```python
from build123d import *

# Parameters (mm, degrees)
SKETCH2_R                            = 2.0193
BOSS_EXTRUDE1_DEPTH                  = 304.8
F_10_32_TAPPED_HOLE2_D               = 4.0386
F_10_32_TAPPED_HOLE2_DEPTH           = 16.34744
F_10_32_TAPPED_HOLE2_TIP             = 1.213317848
F_10_32_TAPPED_HOLE2_ON_FACE_2_D     = 4.0386
F_10_32_TAPPED_HOLE2_ON_FACE_2_DEPTH = 16.34744
F_10_32_TAPPED_HOLE2_ON_FACE_2_TIP   = 1.213317848


with BuildPart() as part:
    # Sketch2 → Boss-Extrude1 (new, symmetric)
    with BuildSketch(Plane.XY):
        with BuildLine():
            ThreePointArc((0.741687758, 5.071047688), (0, 5.125000037), (-0.741687758, 5.071047688))
            Line((-0.741687758, 5.071047688), (-4.020812242, 3.177844283))
            ThreePointArc((-4.020812242, 3.177844283), (-4.438380226, 2.562500019), (-4.7625, 1.893203404))
            Line((-4.7625, 1.893203404), (-4.7625, -1.893203404))
            ThreePointArc((-4.7625, -1.893203404), (-4.438380226, -2.562500019), (-4.020812242, -3.177844283))
            Line((-4.020812242, -3.177844283), (-0.741687758, -5.071047688))
            ThreePointArc((-0.741687758, -5.071047688), (0, -5.125000037), (0.741687758, -5.071047688))
            Line((0.741687758, -5.071047688), (4.020812242, -3.177844283))
            ThreePointArc((4.020812242, -3.177844283), (4.438380226, -2.562500019), (4.7625, -1.893203404))
            Line((4.7625, -1.893203404), (4.7625, 1.893203404))
            ThreePointArc((4.7625, 1.893203404), (4.438380226, 2.562500019), (4.020812242, 3.177844283))
            Line((4.020812242, 3.177844283), (0.741687758, 5.071047688))
        make_face()
        with Locations(Location((0, 0, 0), (0, 0, 180))):
            Circle(SKETCH2_R, mode=Mode.SUBTRACT)
    extrude(amount=BOSS_EXTRUDE1_DEPTH, both=True)

    # #10-32 Tapped Hole2
    with Locations(Plane(origin=(0, 0, -304.8), x_dir=(-1, 0, 0), z_dir=(0, 0, -1))):
        with Locations((0, 0)):
            Hole(F_10_32_TAPPED_HOLE2_D / 2, depth=F_10_32_TAPPED_HOLE2_DEPTH)
            with Locations((0, 0, -(F_10_32_TAPPED_HOLE2_DEPTH + F_10_32_TAPPED_HOLE2_TIP / 2))):  # 118° drill point
                Cone(0, F_10_32_TAPPED_HOLE2_D / 2, F_10_32_TAPPED_HOLE2_TIP, mode=Mode.SUBTRACT)

    # #10-32 Tapped Hole2 on face 2
    with Locations(Plane(origin=(0, 0, 304.8), x_dir=(-1, 0, 0), z_dir=(0, 0, -1))):
        with Locations((0, 0)):
            Hole(F_10_32_TAPPED_HOLE2_ON_FACE_2_D / 2, depth=F_10_32_TAPPED_HOLE2_ON_FACE_2_DEPTH)
            with Locations((0, 0, -(F_10_32_TAPPED_HOLE2_ON_FACE_2_DEPTH + F_10_32_TAPPED_HOLE2_ON_FACE_2_TIP / 2))):  # 118° drill point
                Cone(0, F_10_32_TAPPED_HOLE2_ON_FACE_2_D / 2, F_10_32_TAPPED_HOLE2_ON_FACE_2_TIP, mode=Mode.SUBTRACT)


solid = part.part
```
Work out the finished part from the listing and answer in its coordinate system (mm). Give positions to 0.01 mm unless a question says otherwise; leave off trailing zeros. Loops run counter-clockwise (first coordinate to the right, second up) from the corner with the lowest first, then second, coordinate; pieces in that order, holes last. Notation, with made-up numbers: M 61.25,57 L 77.25,57 A35 cw 77.25,89 Z; hole C 61,-21 d1. An arc over 180 degrees is marked long. One line per item, written item: value. Start each with the question number.
1. Find section B-B (y = 0). Give the vertices of the cut face in (x, z), and give its area (3 significant figures).
2. Each of these flat-tipped pins is pushed along its axis until it touches: P1, Ø3.5, axis at x = 0, y = 0, coming from the +Z side; P2, Ø5, axis at x = -0.5, y = -0.5, coming from the +Z side; P3, Ø2, axis at x = -2.5, z = 242.5, coming from the +Y side; P4, Ø1, axis at y = -3.5, z = -185, coming from the -X side. Where does it stop, or does it pass through?
3. Find the intervals of material crossed by probe 1 along Y at (x, z) = (-0.5, -76); probe 2 along X at (y, z) = (-0.75, 113); probe 3 along Y at (x, z) = (2.75, 267.5), in increasing order.
Reported:
1. outline: M -4.76,-304.8 L -2.02,-304.8 L -2.02,304.8 L -4.76,304.8 Z; M 2.02,-304.8 L 4.76,-304.8 L 4.76,304.8 L 2.02,304.8 Z
1. area: 3,340 mm²
2. P1: passes through
2. P2: stops at z = 304.8
2. P3: stops at y = 4.63
2. P4: stops at x = -4.16
3. probe 1: y = -5.1 to -1.96, 1.96 to 5.1
3. probe 2: x = -4.76 to -1.87, 1.87 to 4.76
3. probe 3: y = -3.91 to 3.91
